from build123d import *

# Parameters (mm, degrees)
SKETCH1_W           = 122
SKETCH1_H           = 102
SKETCH1_W_2         = 110
SKETCH1_H_2         = 90
BOSS_EXTRUDE1_DEPTH = 70
SKETCH3_W           = 10
SKETCH3_H           = 102
BOSS_EXTRUDE3_DEPTH = 122
SKETCH6_R           = 1.5
CUT_EXTRUDE1_DEPTH  = 10
SKETCH5_R           = 1.5
CUT_EXTRUDE2_DEPTH  = 10
SKETCH5_3_R         = 1.5
CUT_EXTRUDE3_DEPTH  = 10
SKETCH8_W           = 5
SKETCH8_H           = 11.8
SKETCH8_H_2         = 11.897582895
BOSS_EXTRUDE4_DEPTH = 22
SKETCH9_R           = 1.5
CUT_EXTRUDE4_DEPTH  = 7
SKETCH10_R          = 1.5
CUT_EXTRUDE5_DEPTH  = 7
SKETCH14_W          = 3
SKETCH14_H          = 6
CUT_EXTRUDE6_DEPTH  = 10


with BuildPart() as part:
    # Sketch1 → Boss-Extrude1 (new body)
    with BuildSketch(Plane.XY):
        Rectangle(SKETCH1_W, SKETCH1_H)
        Rectangle(SKETCH1_W_2, SKETCH1_H_2, mode=Mode.SUBTRACT)
    extrude(amount=BOSS_EXTRUDE1_DEPTH)

    # Sketch3 → Boss-Extrude3 (add)
    with BuildSketch(Plane(origin=(61, 0, 0), x_dir=(0, 0, -1), z_dir=(1, 0, 0))):
        with Locations((-5, 0)):
            Rectangle(SKETCH3_W, SKETCH3_H)
    extrude(amount=-BOSS_EXTRUDE3_DEPTH)

    # Sketch6 → Cut-Extrude1 (cut)
    with BuildSketch(Plane.ZY.offset(61)):
        with Locations((18.78, -31.5)):
            Circle(SKETCH6_R)
        with Locations((46.72, -31.5)):
            Circle(SKETCH6_R)
    extrude(amount=-CUT_EXTRUDE1_DEPTH, mode=Mode.SUBTRACT)

    # Sketch5 → Cut-Extrude2 (cut)
    with BuildSketch(Plane.ZY.offset(61)):
        with Locations((61.96, 19.26)):
            Circle(SKETCH5_R)
    extrude(amount=-CUT_EXTRUDE2_DEPTH, mode=Mode.SUBTRACT)

    # Sketch5_3 → Cut-Extrude3 (cut)
    with BuildSketch(Plane.ZY.offset(61)):
        with Locations((13.7, 19.26)):
            Circle(SKETCH5_3_R)
    extrude(amount=-CUT_EXTRUDE3_DEPTH, mode=Mode.SUBTRACT)

    # Sketch8 → Boss-Extrude4 (add)
    with BuildSketch(Plane.XZ.offset(51)):
        with Locations((18.5, 52.1)):
            Rectangle(SKETCH8_W, SKETCH8_H)
        with Locations((-8.7, 52.051208553)):
            Rectangle(SKETCH8_W, SKETCH8_H_2)
    extrude(amount=-BOSS_EXTRUDE4_DEPTH)

    # Sketch9 → Cut-Extrude4 (cut)
    with BuildSketch(Plane(origin=(0, -17, 0), x_dir=(1, 0, 0), z_dir=(0, 1, 0))):
        with Locations((27.78366931, -52.019097091)):
            Circle(SKETCH9_R)
    extrude(amount=-CUT_EXTRUDE4_DEPTH, mode=Mode.SUBTRACT)

    # Sketch10 → Cut-Extrude5 (cut)
    with BuildSketch(Plane(origin=(0, -17, 0), x_dir=(1, 0, 0), z_dir=(0, 1, 0))):
        with Locations((2.714757204, -51.901428217)):
            Circle(SKETCH10_R)
    extrude(amount=-CUT_EXTRUDE5_DEPTH, mode=Mode.SUBTRACT)

    # Sketch14 → Cut-Extrude6 (cut)
    with BuildSketch(Plane.ZY.offset(11.2)):
        with Locations((52.1, -42)):
            Rectangle(SKETCH14_W, SKETCH14_H)
    extrude(amount=-CUT_EXTRUDE6_DEPTH, mode=Mode.SUBTRACT)


solid = part.part
Verification items for the finished model (mm, model axes). A direction names the side the tool comes from. Coordinates: 2 decimals unless noted, no trailing zeros. Order: outer loops, then holes, each group sorted by start corner. A loop starts at its lowest first (then second) coordinate and runs counter-clockwise, first axis right, second up. Notation, with made-up numbers: M 87,44.5 L 92,44.5 A18 cw 92,63.5 Z; hole C -32,17 d9. An arc over 180 degrees is marked long. One line per item, written item: value. Start each with the question number.
Item 1: Sectioned sample at D-D (x = -52). Enter the section's corners in (y, z), then the cut area to 3 significant figures.
Item 2: Sectioned sample at B-B (y = 19.26). Enter the section's corners in (x, z).
Item 3: Sectioned sample at C-C (z = 36.5). Enter the section's corners in (x, y), then the cut area to 3 significant figures.
Item 4: Access from +Z, -Z, +X, -X, +Y, -Y to the whole of each face (thin tool, end or side, straight path). Record for faces 4 (the cylindrical face through (-58.042, -30.013, 18.585)), 5 (the flat face through (-9, -42, 50.6)), 6 (the flat face through (18, -29, 52)).
Item 5: Mould release check, pull along Y, two halves, no side actions. Record for faces 1 (the flat face through (61, -1, 35)), 2 (the flat face through (-9, -42, 53.6)), 3 (the flat face through (21, -37, 52)): released by +Y, released by -Y, zero draft, split by the parting line, or undercut.
Item 6: Sectioned sample at A-A (y = -31.5). Enter the section's corners in (x, z), then the cut area to 3 significant figures.
Item 7: Scan lines: probe 1 along Y at (x, z) = (-58.9, 18.78); probe 2 along X at (y, z) = (17, 35); probe 3 along Z at (x, y) = (-58, -31). Record each from-to range of solid material in increasing order.
Item 8: Gauge pin test, flat ends, axial feed: pin 1 (4 mm diameter, centred on x = -33.5, y = 34.5, fed in from +Z); pin 2 (5.5 mm diameter, centred on x = -8.5, y = -36.5, fed in from +Z); pin 3 (2.5 mm diameter, centred on x = -8, y = -41, fed in from -Z). Record the tip position at first contact, or that the pin passes through.
Conclusion:
1. outline: M -51,0 L 51,0 L 51,70 L 45,70 L 45,10 L -45,10 L -45,70 L -51,70 Z
1. area: 1,740 mm^2
2. outline: M -61,0 L 61,0 L 61,70 L 55,70 L 55,10 L -55,10 L -55,12.2 L -61,12.2 Z; M -61,15.2 L -55,15.2 L -55,60.46 L -61,60.46 Z; M -61,63.46 L -55,63.46 L -55,70 L -61,70 Z
3. outline: M -61,-51 L 61,-51 L 61,51 L -61,51 Z; hole M -55,-45 L 55,-45 L 55,45 L -55,45 Z
3. area: 2,540 mm^2
4. face 4: -X
4. face 5: none
4. face 6: +Z
5. face 1: zero draft
5. face 2: undercut
5. face 3: undercut
6. outline: M -61,0 L 61,0 L 61,70 L 55,70 L 55,10 L -55,10 L -55,17.28 L -61,17.28 Z; M -61,20.28 L -55,20.28 L -55,45.22 L -61,45.22 Z; M -61,48.22 L -55,48.22 L -55,70 L -61,70 Z; M -11.2,46.1 L -6.2,46.1 L -6.2,58 L -11.2,58 Z; M 16,46.2 L 21,46.2 L 21,58 L 16,58 Z
6. area: 2,020 mm^2
7. probe 1: y = -51 to -33, -30 to 51
7. probe 2: x = -61 to -55, 55 to 61
7. probe 3: z = 0 to 17.37, 20.19 to 45.31, 48.13 to 70
8. pin 1: stops at z = 10
8. pin 2: stops at z = 58
8. pin 3: stops at z = 0
